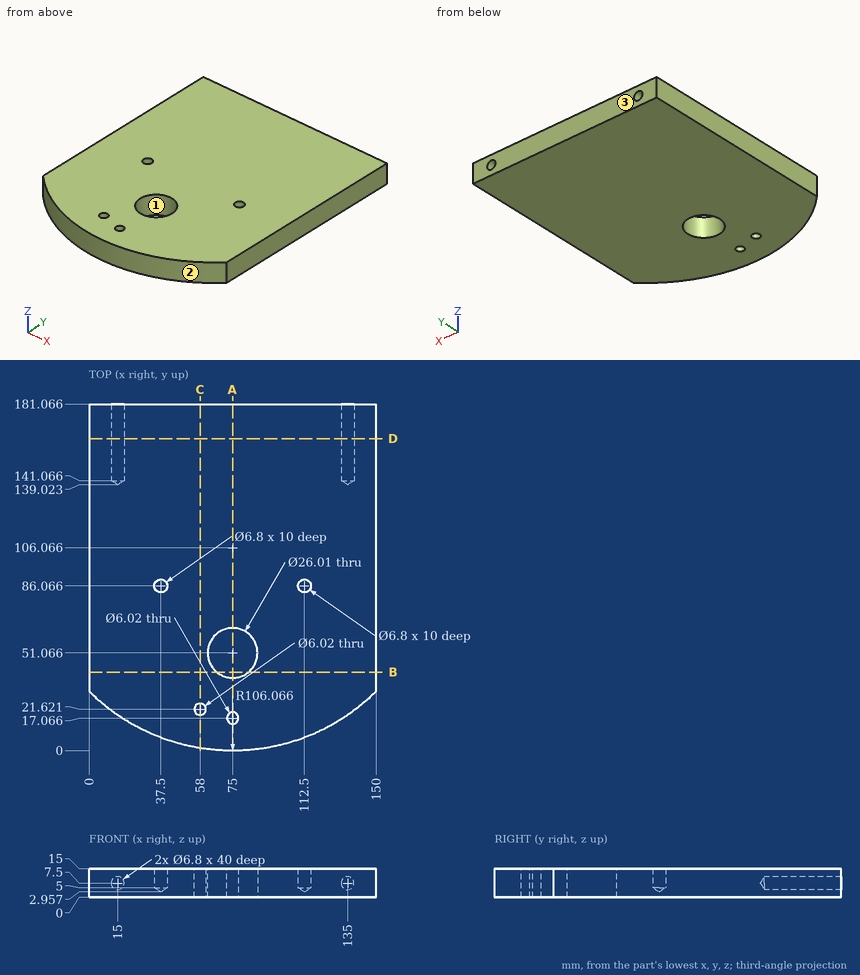
Source: three-view drawing plus pictorial views. Frame: mm from the lowest corner of the part. Round coordinates to 2 decimals unless told otherwise and drop trailing zeros. Loops run counter-clockwise (first coordinate to the right, second up) from the corner with the lowest first, then second, coordinate; pieces in that order, holes last. Notation, with made-up numbers: M -35.75,18.5 L 21.25,18.5 A9 cw 21.25,31.5 Z; hole C 88,80 d11. An arc over 180 degrees is marked long. Answer as CSV lines item,"result".
Q1. Cut plane D-D (y = 163). Return the cut outline in (x, z), plus the area to 3 significant figures.
Verdict:
outline,"M 0,0 L 150,0 L 150,15 L 0,15 Z; hole C 15,7.5 d6.8; hole C 135,7.5 d6.8"
area,"2,180 mm^2"
Q2. Contact query for flat-ended pins moving along their axis: pin 1 (4 mm diameter, centred on x = 15, z = 7.5, fed in from -Y); pin 2 (6 mm diameter, centred on x = 135, z = 7.5, fed in from -Y); pin 3 (3.5 mm diameter, centred on x = 58, y = 21.62, fed in from +Z). Output: stop coordinate, or through.
Verdict:
pin 1,"stops at y = 17.26"
pin 2,"stops at y = 16.62"
pin 3,"passes through"
Q3. Cut plane C-C (x = 58). Return the cut outline in (y, z), plus the area to 4 significant figures.
Verdict:
outline,"M 1.37,0 L 18.61,0 L 18.61,15 L 1.37,15 Z; M 24.63,0 L 181.07,0 L 181.07,15 L 24.63,15 Z"
area,"2,605 mm^2"
Q4. Cut plane A-A (x = 75). Return the cut outline in (y, z).
Verdict:
outline,"M 0,0 L 14.06,0 L 14.06,15 L 0,15 Z; M 20.08,0 L 38.06,0 L 38.06,15 L 20.08,15 Z; M 64.07,0 L 181.07,0 L 181.07,15 L 64.07,15 Z"
Q5. Cut plane B-B (y = 41). Return the cut outline in (x, z).
Verdict:
outline,"M 0,0 L 66.77,0 L 66.77,15 L 0,15 Z; M 83.23,0 L 150,0 L 150,15 L 83.23,15 Z"
Q6. Pull-direction query (X, two-part tool) for the marked faces 1, 2 and 3; classes: +X half, -X half, draft (parallel to the pull), parting line (faces both ways), or undercut.
Verdict:
face 1,"undercut"
face 2,"parting line"
face 3,"draft"
Q7. Line query: line 1 along Z through (x, y) = (135, 164.5); line 2 along Y through (x, z) = (73, 6.75) (1 decimal); line 3 along Y through (x, z) = (67, 7). Output: solid intervals per line, ascending.
Verdict:
line 1,"z = 0 to 4.1, 10.9 to 15"
line 2,"y = 0 to 14.8, 19.3 to 38.2, 63.9 to 181.1"
line 3,"y = 0.3 to 40.81, 61.32 to 181.07"
